The model under review builds one solid part; all positions refer to its coordinate system, in mm. Give positions to 0.01 mm unless a question says otherwise; leave off trailing zeros. Order: outer loops, then holes, each group sorted by start corner. A loop starts at its lowest first (then second) coordinate and runs counter-clockwise, first axis right, second up. Notation, with made-up numbers: (11, 26) - (27, 26) arc R13 ccw to (27, 36) - close; hole circle Ø7 at (81, 22.25). An arc over 180 degrees is marked (long way). Use CSV: the item, a comma, the result in double quotes.
Autodesk Inventor part; units mm, degrees
ref_plane "YZ Plane" through (0, 0, 0) normal (1, 0, 0) x (0, 1, 0)
ref_plane "XZ Plane" through (0, 0, 0) normal (0, 1, 0) x (-1, 0, 0)
ref_plane "XY Plane" through (0, 0, 0) normal (0, 0, 1) x (1, 0, 0)
sketch "Sketch1" plane through (0, 0, 0) normal (0, 1, 0) x (-1, 0, 0)
  line L0 (-25.4, -38.1) -> (25.4, -38.1) construction
  line L1 (25.4, -38.1) -> (25.4, -29.8901)
  line L2 (25.4, 38.1) -> (-25.4, 38.1) construction
  line L3 (-25.4, -29.8901) -> (-25.4, -38.1)
  line L4 (-25.4, -38.1) -> (25.4, 38.1) construction
  line L5 (25.4, -38.1) -> (-25.4, 38.1) construction
  circle A0 centre (12.7, -28.575) radius 4.7625
  circle A1 centre (0, -28.575) radius 4.7625
  circle A2 centre (-12.7, -28.575) radius 4.7625
  circle A3 centre (12.7, -15.875) radius 4.7625
  circle A4 centre (0, -15.875) radius 4.7625
  circle A5 centre (-12.7, -15.875) radius 4.7625
  circle A6 centre (12.7, -3.175) radius 4.7625
  circle A7 centre (0, -3.175) radius 4.7625
  circle A8 centre (-12.7, -3.175) radius 4.7625
  circle A9 centre (12.7, 9.525) radius 4.7625
  circle A10 centre (0, 9.525) radius 4.7625
  circle A11 centre (-12.7, 9.525) radius 4.7625
  circle A12 centre (12.7, 22.225) radius 4.7625
  circle A13 centre (0, 22.225) radius 4.7625
  circle A14 centre (-12.7, 22.225) radius 4.7625
  line L6 (47.625, -15.875) -> (47.625, 9.525) construction
  circle A15 centre (25.4, -3.175) radius 4.7625
  circle A16 centre (38.1, -3.175) radius 4.7625
  line L7 (0, -38.1) -> (0, 38.1) construction
  circle A17 centre (-25.4, -3.175) radius 4.7625
  circle A18 centre (-38.1, -3.175) radius 4.7625
  arc A19 (39.4151, -15.875) -> (25.4, -29.8901) centre (39.4151, -29.8901) ccw construction
  line L8 (25.4, 38.1) -> (25.4, 23.5401) construction
  arc A20 (25.4, 23.5401) -> (39.4151, 9.525) centre (39.4151, 23.5401) ccw construction
  line L9 (-60.325, -15.875) -> (-39.4151, -15.875) construction
  line L10 (-60.325, 9.525) -> (-39.4151, 9.525) construction
  arc A21 (-25.4, -29.8901) -> (-39.4151, -15.875) centre (-39.4151, -29.8901) ccw construction
  line L11 (-25.4, 23.5401) -> (-25.4, 38.1) construction
  arc A22 (-39.4151, 9.525) -> (-25.4, 23.5401) centre (-39.4151, 23.5401) ccw construction
  line L12 (53.975, -15.875) -> (28.575, -15.875) construction
  line L13 (25.4, -19.05) -> (25.4, -44.45) construction
  line L14 (-25.4, -44.45) -> (-25.4, -19.05) construction
  line L15 (-28.575, -15.875) -> (-39.4151, -15.875) construction
  line L16 (-25.4, 23.5401) -> (-25.4, 12.7) construction
  line L17 (-39.4151, 9.525) -> (-28.575, 9.525) construction
  line L18 (25.4, 23.5401) -> (25.4, 12.7) construction
  line L19 (28.575, 9.525) -> (53.975, 9.525) construction
  arc A23 (25.4, 12.7) -> (28.575, 9.525) centre (28.575, 12.7) ccw construction
  arc A24 (28.575, -15.875) -> (25.4, -19.05) centre (28.575, -19.05) ccw construction
  arc A25 (-25.4, -19.05) -> (-28.575, -15.875) centre (-28.575, -19.05) ccw construction
  arc A26 (-28.575, 9.525) -> (-25.4, 12.7) centre (-28.575, 12.7) ccw construction
  line L20 (39.4151, -22.225) -> (53.975, -22.225)
  line L21 (53.975, -22.225) -> (53.975, 15.875) construction
  line L22 (53.975, 15.875) -> (39.4151, 15.875)
  arc A27 (39.4151, -22.225) -> (31.75, -29.8901) centre (39.4151, -29.8901) ccw
  line L23 (31.75, -29.8901) -> (31.75, -44.45)
  line L24 (31.75, -44.45) -> (-31.75, -44.45) construction
  line L25 (-31.75, -44.45) -> (-31.75, -29.8901)
  arc A28 (-31.75, -29.8901) -> (-39.4151, -22.225) centre (-39.4151, -29.8901) ccw
  line L26 (-39.4151, -22.225) -> (-60.325, -22.225)
  line L27 (-60.325, -22.225) -> (-60.325, 15.875)
  line L28 (-60.325, 15.875) -> (-39.4151, 15.875)
  arc A29 (-39.4151, 15.875) -> (-31.75, 23.5401) centre (-39.4151, 23.5401) ccw
  line L29 (-31.75, 23.5401) -> (-31.75, 44.45)
  line L30 (-31.75, 44.45) -> (31.75, 44.45)
  line L31 (31.75, 44.45) -> (31.75, 23.5401)
  arc A30 (31.75, 23.5401) -> (39.4151, 15.875) centre (39.4151, 23.5401) ccw
  line L32 (25.4, 38.1) -> (25.4, 44.45) construction
  line L33 (-25.4, 38.1) -> (-25.4, 44.45)
  circle A31 centre (-55.5625, -3.175) radius 4.7625 construction
  circle A32 centre (49.2125, -3.175) radius 4.7625 construction
  circle A33 centre (0, -39.6875) radius 4.7625 construction
  circle A34 centre (0, 39.6875) radius 4.7625 construction
  line L34 (44.45, -17.4132) -> (44.45, -3.2681) construction
  line L35 (-50.8, -20.963) -> (-50.8, -1.2168) construction
  line L36 (-5.6388, -34.925) -> (9.5526, -34.925) construction
  line L37 (-7.9375, 34.925) -> (9.5526, 34.925) construction
  circle A35 centre (-55.5625, -3.175) radius 2.4892 construction
  circle A36 centre (0, -39.6875) radius 2.4892 construction
  circle A37 centre (49.2125, -3.175) radius 2.4892
  circle A38 centre (0, 39.6875) radius 2.4892 construction
  line L38 (33.9951, -24.4701) -> (26.3299, -16.8049) construction
  circle A39 centre (30.1625, -20.6375) radius 2.5527
  circle A40 centre (-30.1625, -20.6375) radius 2.5527
  line L39 (53.975, -3.175) -> (-60.325, -3.175) construction
  circle A41 centre (30.1625, 14.2875) radius 2.5527
  circle A42 centre (-30.1625, 14.2875) radius 2.5527
  circle A43 centre (25.4, 39.6875) radius 2.4892
  circle A44 centre (12.7, 39.6875) radius 2.4892 construction
  circle A45 centre (0, 39.6875) radius 2.4892 construction
  circle A46 centre (-12.7, 39.6875) radius 2.4892 construction
  circle A47 centre (-25.4, 39.6875) radius 2.4892
  circle A48 centre (12.7, -39.6875) radius 2.4892
  circle A49 centre (25.4, -39.6875) radius 2.4892 construction
  circle A50 centre (-12.7, -39.6875) radius 2.4892
  circle A51 centre (-25.4, -39.6875) radius 2.4892 construction
  circle A52 centre (49.2125, -11.1125) radius 2.4892 construction
  circle A53 centre (30.1625, -20.6375) radius 4.7625 construction
  circle A54 centre (49.2125, 4.7625) radius 2.4892 construction
  circle A55 centre (49.2125, 4.7625) radius 4.7625 construction
  circle A56 centre (49.2125, -11.1125) radius 4.7625 construction
  circle A57 centre (-55.5625, -11.1125) radius 2.4892
  circle A58 centre (-55.5625, -11.1125) radius 4.7625 construction
  circle A59 centre (-55.5625, 4.7625) radius 2.4892
  circle A60 centre (-55.5625, 4.7625) radius 4.7625 construction
  circle A61 centre (-12.7, 33.3375) radius 2.4892
  circle A62 centre (12.7, 33.3375) radius 2.4892
  circle A63 centre (-25.4, -46.0375) radius 2.4892
  circle A64 centre (25.4, -46.0375) radius 2.4892
  line L40 (31.75, -44.45) -> (31.75, -50.8)
  line L41 (31.75, -50.8) -> (-31.75, -50.8)
  line L42 (-31.75, -50.8) -> (-31.75, -44.45)
  line L43 (25.4, -44.45) -> (25.4, -50.8) construction
  line L44 (-25.4, -44.45) -> (-25.4, -50.8) construction
  circle A65 centre (-49.2125, -3.175) radius 2.4892
  circle A66 centre (55.5625, 4.7625) radius 2.4892
  circle A67 centre (55.5625, -11.1125) radius 2.4892
  line L45 (53.975, -22.225) -> (60.325, -22.225)
  line L46 (60.325, -22.225) -> (60.325, 15.875)
  line L47 (53.975, 15.875) -> (60.325, 15.875)
  line L48 (53.975, 9.525) -> (60.325, 9.525) construction
  line L49 (53.975, -15.875) -> (60.325, -15.875) construction
  circle A68 centre (25.4, -46.0375) radius 4.7625
  line L50 (25.4, -41.275) -> (19.287, -41.275)
  circle A69 centre (12.7, 33.3375) radius 4.7625
  line L51 (15.952, 28.575) -> (5.0903, 28.575) construction
  circle A70 centre (55.5625, 4.7625) radius 4.7625 construction
  line L52 (50.8, 8.631) -> (50.8, -0.466) construction
  point P0 (0, 0)
  point P1 (47.625, -3.175)
  point P2 (-25.4, 9.525)
  point P3 (47.625, -15.875)
  point P4 (47.625, 9.525)
  dimension "d15" = 25.4
  dimension "d0" = 50.8
  dimension "d3" = 9.525
  dimension "d6" = 12.7
  dimension "d9" = 12.7
  dimension "d18" = 12.7
  dimension "d29" = 3.175
  dimension "d30" = 6.35
  dimension "d31" = 7.6651
  dimension "d65" = 9.525
  dimension "d67" = 6.35
  dimension "d68" = 12.7
  dimension "d69" = 4.7625
  dimension "d70" = 25.4
  dimension "d71" = 6.35
  dimension "d74" = 12.7
  dimension "d89" = 4.9784
  dimension "d90" = 5.1054
  dimension "d100" = 4.9784
  dimension "d101" = 6.35
  dimension "d104" = 12.7
  dimension "d112" = 360
  dimension "d114" = 4.9784
  dimension "d126" = 9.525
  dimension "d127" = 9.525
  dimension "d128" = 9.525
  dimension "d129" = 4.9784
  dimension "d132" = 360
  dimension "d134" = 47.625
  dimension "d135" = 47.625
  dimension "d138" = 360
  dimension "d140" = 60.325
  dimension "d141" = 60.325
  dimension "d142" = 6.35
  dimension "d143" = 12.7
extrude "Extrusion1" add sketch "Sketch1" along normal blind 6.35 contours A68 | A27 L23 L40 L41 L42 L25 A28 L26 L27 L28 A29 L29 L30 L31 A30 L22 L47 L46 L45 L20 | A69
sketch "Sketch2" plane through (0, 0, 0) normal (0, -1, 0) x (1, 0, 0)
  circle A0 centre (38.1, -3.175) radius 4.7625
  circle A1 centre (25.4, -3.175) radius 4.7625
  circle A2 centre (12.7, -28.575) radius 4.7625
  circle A3 centre (12.7, -15.875) radius 4.7625
  circle A4 centre (12.7, -3.175) radius 4.7625
  circle A5 centre (12.7, 9.525) radius 4.7625
  circle A6 centre (12.7, 22.225) radius 4.7625
  circle A7 centre (0, 22.225) radius 4.7625
  circle A8 centre (-12.7, 22.225) radius 4.7625
  circle A9 centre (-25.4, -3.175) radius 4.7625
  circle A10 centre (-38.1, -3.175) radius 4.7625
  circle A11 centre (-12.7, 9.525) radius 4.7625
  circle A12 centre (0, 9.525) radius 4.7625
  circle A13 centre (0, -28.575) radius 4.7625
  circle A14 centre (-12.7, -28.575) radius 4.7625
  circle A15 centre (0, -15.875) radius 4.7625
  circle A16 centre (-12.7, -15.875) radius 4.7625
  circle A17 centre (0, -3.175) radius 4.7625
  circle A18 centre (-12.7, -3.175) radius 4.7625
  point P0 (0, 0)
  point P1 (38.1, -3.175)
  point P2 (25.4, -3.175)
  point P3 (12.7, -28.575)
  point P4 (12.7, -15.875)
  point P5 (12.7, -3.175)
  point P6 (12.7, 9.525)
  point P7 (12.7, 22.225)
  point P8 (0, 22.225)
  point P9 (-12.7, 22.225)
  point P10 (-25.4, -3.175)
  point P11 (-38.1, -3.175)
  point P12 (-12.7, 9.525)
  point P13 (0, 9.525)
  point P14 (0, -28.575)
  point P15 (-12.7, -28.575)
  point P16 (0, -15.875)
  point P17 (-12.7, -15.875)
  point P18 (0, -3.175)
  point P19 (-12.7, -3.175)
hole "Hole1" at (38.1, 0, -3.175) at (25.4, 0, -3.175) at (12.7, 0, -28.575) at (12.7, 0, -15.875) at (12.7, 0, -3.175) at (12.7, 0, 9.525) at (12.7, 0, 22.225) at (0, 0, 22.225) at (-12.7, 0, 22.225) at (-25.4, 0, -3.175) at (-38.1, 0, -3.175) at (-12.7, 0, 9.525) at (0, 0, 9.525) at (0, 0, -28.575) at (-12.7, 0, -28.575) at (0, 0, -15.875) at (-12.7, 0, -15.875) at (0, 0, -3.175) at (-12.7, 0, -3.175) direction (0, 1, 0) diameter 9.525 depth 9.525 counterbore diameter 11.9888 counterbore depth 1.524
fillet "Fillet1" radius 3.175 8 edges at (-31.75, 3.175, 44.45) (60.325, 3.175, 15.875) (31.75, 3.175, 44.45) (60.325, 3.175, -22.225) (-31.75, 3.175, -50.8) (31.75, 3.175, -50.8) (-60.325, 3.175, 15.875) (-60.325, 3.175, -22.225)
equation "\"adder\" = d30"
properties part number "Drill Guide" material "Aluminum 6061"
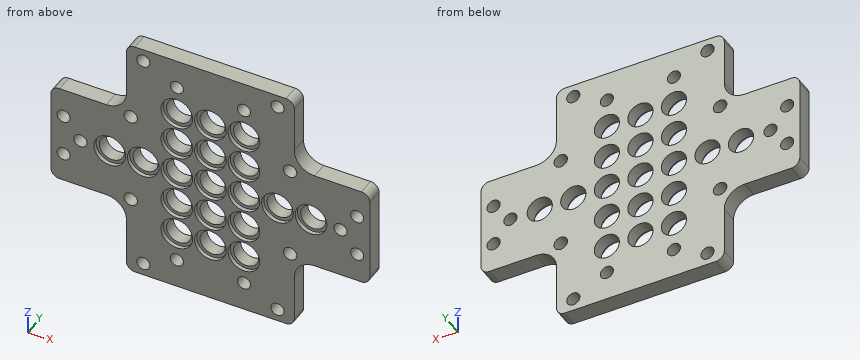
Item 1: Take a section at A-A, the plane x = 25.4. Give the boundary of the cut face in (y, z).
Results list:
outline,"(0, -50.8) - (6.35, -50.8) - (6.35, -48.53) - (0, -48.53) - close; (0, -43.55) - (6.35, -43.55) - (6.35, -7.94) - (1.52, -7.94) - (1.52, -9.17) - (0, -9.17) - close; (0, 2.82) - (1.52, 2.82) - (1.52, 1.59) - (6.35, 1.59) - (6.35, 37.2) - (0, 37.2) - close; (0, 42.18) - (6.35, 42.18) - (6.35, 44.45) - (0, 44.45) - close"
Item 2: Take a section at B-B, the plane x = 38.1. Give the boundary of the cut face in (y, z).
Results list:
outline,"(0, -22.34) - (6.35, -22.34) - (6.35, -7.94) - (1.52, -7.94) - (1.52, -9.17) - (0, -9.17) - close; (0, 2.82) - (1.52, 2.82) - (1.52, 1.59) - (6.35, 1.59) - (6.35, 15.99) - (0, 15.99) - close"
Item 3: Clearance check with flat-ended pins moving along their axes: pin 1 (4.5 mm diameter, centred on x = -25.4, z = 39.69, fed in from +Y); pin 2 (4 mm diameter, centred on x = -25.5, z = 22, fed in from -Y); pin 3 (3 mm diameter, centred on y = 3.5, z = 16.5, fed in from +X); pin 4 (2 mm diameter, centred on y = 5.5, z = 34.5, fed in from +X). State where each tip first meets the part, or that it passes through.
Results list:
pin 1,"passes through"
pin 2,"stops at y = 0"
pin 3,"stops at x = 59.34"
pin 4,"stops at x = 31.75"
Item 4: Wall thickness on L1, parallel to X at y = 5.25, z = -11.5 (3 decimals); L2, parallel to X at y = 4, z = -10.5 (3 decimals); L3, parallel to X at y = 5.5, z = -38: over which ranges is each line inside the solid? List them lowest first.
Results list:
L1,"x = -60.325 to -58.021, -53.104 to -14.582, -10.818 to -1.882, 1.882 to 10.818, 14.582 to 53.104, 58.021 to 60.325"
L2,"x = -60.325 to -57.975, -53.15 to 53.15, 57.975 to 60.325"
L3,"x = -31.75 to -14.53, -10.87 to 10.87, 14.53 to 31.75"
Item 5: Take a section at C-C, the plane x = 0. State how many separate pieces and enclosed holes the cut face has, and give its area (3 significant figures).
Results list:
separate pieces,"6"
enclosed holes,"0"
area,"284 mm2"
